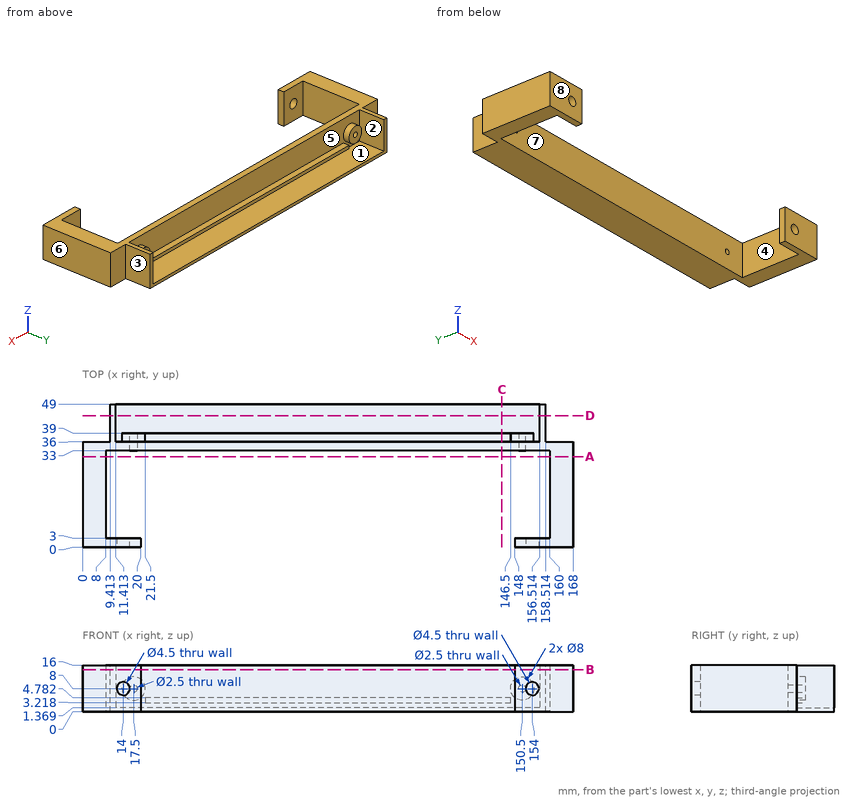
Check sheet for the drawn part. Datum: minimum x, y, z corner. Units: mm. A direction names the side the tool comes from. Coordinates: 2 decimals unless noted, no trailing zeros. Loops run counter-clockwise (first coordinate to the right, second up) from the corner with the lowest first, then second, coordinate; pieces in that order, holes last. Notation, with made-up numbers: (4.5, -5.75) -> (9.5, -5.75) arc R30 ccw to (9.5, 20.25) -> close; hole circle Ø11 at (2.5, -15.5). An arc over 180 degrees is marked (long way). Answer in a Markdown table with one row per item.
1) Depth check by flat-ended pin: P1, Ø4, axis at x = 154, z = 8, coming from the -Y side; P2, Ø4, axis at x = 20.5, z = 14.5, coming from the +Y side; P3, Ø2.5, axis at x = 18.5, z = 9, coming from the +Y side. Enter the tip coordinate at first touch or a pass-through.
The answers:
| item | result |
|---|---|
| P1 | stops at y = 33 |
| P2 | stops at y = 36 |
| P3 | stops at y = 39 |
2) Section check A-A (y = 31). Record the cut outline in (x, z), and give its area (3 significant figures).
The answers:
| item | result |
|---|---|
| outline | (0, 0) -> (8, 0) -> (8, 16) -> (0, 16) -> close; (160, 0) -> (168, 0) -> (168, 16) -> (160, 16) -> close |
| area | 256 mm2 |
3) Section check C-C (x = 143.5). Record the cut outline in (y, z).
The answers:
| item | result |
|---|---|
| outline | (33, 0) -> (49, 0) -> (49, 1.37) -> (36, 1.37) -> (36, 3.22) -> (39, 3.22) -> (39, 4.78) -> (36, 4.78) -> (36, 16) -> (33, 16) -> close |
4) Scan lines: line 1 along Z through (x, y) = (17.5, 36.9); line 2 along X through (y, z) = (36.15, 8); line 3 along X through (y, z) = (34.6, 8). Record each from-to range of solid material in increasing order. Write a range as from..to.
The answers:
| item | result |
|---|---|
| line 1 | z = 0..1.37, 4..6.75, 9.25..12 |
| line 2 | x = 9.41..11.41, 13.5..16.25, 18.75..21.5, 146.5..149.25, 151.75..154.5, 156.51..158.51 |
| line 3 | x = 0..16.25, 18.75..149.25, 151.75..168 |
5) Access from +Z, -Z, +X, -X, +Y, -Y to the whole of each face (thin tool, end or side, straight path). Record for the marked faces 1, 2, 3 and 4.
The answers:
| item | result |
|---|---|
| face 1 | +Y |
| face 2 | +Z, +Y |
| face 3 | +Z, -Z, +X, +Y |
| face 4 | +Z, -Z |
6) Draft check along X on the marked faces 5, 6, 7 and 8. Enter one of: released by +X, released by -X, zero draft, split by the parting line, or undercut.
The answers:
| item | result |
|---|---|
| face 5 | undercut |
| face 6 | released by +X |
| face 7 | undercut |
| face 8 | zero draft |
7) Section check B-B (z = 14.5). Record the cut outline in (x, y).
The answers:
| item | result |
|---|---|
| outline | (0, 0) -> (20, 0) -> (20, 3) -> (8, 3) -> (8, 33) -> (160, 33) -> (160, 3) -> (148, 3) -> (148, 0) -> (168, 0) -> (168, 36) -> (158.51, 36) -> (158.51, 49) -> (156.51, 49) -> (156.51, 36) -> (11.41, 36) -> (11.41, 49) -> (9.41, 49) -> (9.41, 36) -> (0, 36) -> close |
8) Section check D-D (y = 45). Record the cut outline in (x, z).
The answers:
| item | result |
|---|---|
| outline | (9.41, 0) -> (158.51, 0) -> (158.51, 16) -> (156.51, 16) -> (156.51, 1.37) -> (11.41, 1.37) -> (11.41, 16) -> (9.41, 16) -> close |
